Design review of the part built by this model. Coordinates are the model's own, in mm. A direction names the side the tool comes from. Give positions to 0.01 mm unless a question says otherwise; leave off trailing zeros. Write each loop counter-clockwise with the first axis right and the second up, starting at its lowest first coordinate (ties: lowest second). Pieces come first, ordered by that corner, then holes. Notation, with made-up numbers: M 67,43 L 90,43 A15 cw 90,60 Z; hole C 77.25,36.5 d6. An arc over 180 degrees is marked long. One line per item, written item: value. Start each with the question number.
```python
from build123d import *

# Parameters (mm, degrees)
SKETCH2_W           = 280
SKETCH2_H           = 12
SKETCH2_R           = 2
BOSS_EXTRUDE1_DEPTH = 4
CUT_EXTRUDE1_DEPTH  = 281
SKETCH5_R           = 2
BOSS_EXTRUDE2_DEPTH = 2
SKETCH4_W           = 18
SKETCH4_H           = 12
CUT_EXTRUDE2_DEPTH  = 9
BOSS_EXTRUDE3_REACH = 10
SKETCH7_R           = 2
SKETCH8_R           = 2
SKETCH8_R_2         = 1.5
BOSS_EXTRUDE4_DEPTH = 2


with BuildPart() as part:
    # Sketch2 → Boss-Extrude1 (new body, symmetric)
    with BuildSketch(Plane(origin=(0, 0, 0), x_dir=(1, 0, 0), z_dir=(0, 1, 0))):
        Rectangle(SKETCH2_W, SKETCH2_H)
        with Locations((-125, 0)):
            Circle(SKETCH2_R, mode=Mode.SUBTRACT)
        with Locations((-75, 0)):
            Circle(SKETCH2_R, mode=Mode.SUBTRACT)
        with Locations((-25, 0)):
            Circle(SKETCH2_R, mode=Mode.SUBTRACT)
        with Locations((25, 0)):
            Circle(SKETCH2_R, mode=Mode.SUBTRACT)
        with Locations((75, 0)):
            Circle(SKETCH2_R, mode=Mode.SUBTRACT)
        with Locations((125, 0)):
            Circle(SKETCH2_R, mode=Mode.SUBTRACT)
    extrude(amount=BOSS_EXTRUDE1_DEPTH, both=True)

    # Sketch3 → Cut-Extrude1 (cut, through all)
    with BuildSketch(Plane.ZY.offset(140)):
        Polygon((-6, 2.625), (-6, 0.375), (-4.5, 1), (-4.5, 2), align=None)
        Polygon((6, 2.625), (6, 0.375), (4.5, 1), (4.5, 2), align=None)
    extrude(amount=-CUT_EXTRUDE1_DEPTH, mode=Mode.SUBTRACT)

    # Sketch5 → Boss-Extrude2 (add)
    with BuildSketch(Plane(origin=(0, 4, 0), x_dir=(1, 0, 0), z_dir=(0, 1, 0))):
        with Locations((-75, 0)):
            Circle(SKETCH5_R)
        with Locations((-25, 0)):
            Circle(SKETCH5_R)
        with Locations((25, 0)):
            Circle(SKETCH5_R)
        with Locations((75, 0)):
            Circle(SKETCH5_R)
        with Locations((-125, 0)):
            Circle(SKETCH5_R)
        with Locations((125, 0)):
            Circle(SKETCH5_R)
    extrude(amount=-BOSS_EXTRUDE2_DEPTH)

    # Sketch4 → Cut-Extrude2 (cut, through all)
    with BuildSketch(Plane(origin=(0, 4, 0), x_dir=(1, 0, 0), z_dir=(0, 1, 0))):
        with Locations((-131, 0)):
            Rectangle(SKETCH4_W, SKETCH4_H)
    cut_extrude2 = extrude(amount=-CUT_EXTRUDE2_DEPTH, mode=Mode.SUBTRACT)

    # Mirror1: Cut-Extrude2 across plane
    add(cut_extrude2.mirror(Plane(origin=(0, 0, 0), x_dir=(0, 0, 1), z_dir=(1, 0, 0))), mode=Mode.SUBTRACT)

    # Sketch7 → Boss-Extrude3 (add, up to next)
    with BuildSketch(Plane.XZ.offset(4), mode=Mode.PRIVATE) as boss_extrude3_sk1:
        with Locations((-75, 0)):
            Circle(SKETCH7_R)
    boss_extrude3_tool1 = extrude(boss_extrude3_sk1.sketch, amount=-BOSS_EXTRUDE3_REACH, mode=Mode.PRIVATE) - part.part
    add(boss_extrude3_tool1.solids().sort_by_distance((-75, -4, 0))[0])
    # Sketch7 → Boss-Extrude3 (add, up to next)
    with BuildSketch(Plane.XZ.offset(4), mode=Mode.PRIVATE) as boss_extrude3_sk2:
        with Locations((75, 0)):
            Circle(SKETCH7_R)
    boss_extrude3_tool2 = extrude(boss_extrude3_sk2.sketch, amount=-BOSS_EXTRUDE3_REACH, mode=Mode.PRIVATE) - part.part
    add(boss_extrude3_tool2.solids().sort_by_distance((75, -4, 0))[0])

    # Sketch8 → Boss-Extrude4 (add)
    with BuildSketch(Plane.XZ.offset(-2)):
        with Locations((-25, 0)):
            Circle(SKETCH8_R)
        with Locations((-25, 0)):
            Circle(SKETCH8_R_2, mode=Mode.SUBTRACT)
        with Locations((25, 0)):
            Circle(SKETCH8_R)
        with Locations((25, 0)):
            Circle(SKETCH8_R_2, mode=Mode.SUBTRACT)
    extrude(amount=BOSS_EXTRUDE4_DEPTH)


solid = part.part
```
Q1. The part is to be moulded in two halves that separate along X. For faces 1 (the face through (-2, -2, -6)), 2 (the face through (122, 0, 0)), 3 (the face through (-27, -2, 0)), say which applies: pulls with the +X half, pulls with the -X half, needs draft (parallel to the pull), parting line crosses it, or undercut.
Q2. Take a section at A-A, the plane x = 57.5. Give the boundary of the cut face in (y, z) (3 decimals).
Q3. For P1, Ø1.2, axis at x = -25, z = -0.5, coming from the -Y side; P2, Ø0.8, axis at x = 60.5, y = 1.5, coming from the +Z side; P3, Ø0.8, axis at x = -39.5, y = 1.5, coming from the -Z side, all flat-tipped, find the tip position at first contact; note any pin that passes through.
Q4. Wall thickness on line 1 (X direction, y = -2, z = 0); line 2 (Z direction, x = -25, y = 1.65); line 3 (Z direction, x = -25, y = -2.2): over which ranges is each line inside the solid? List them lowest first. Write a range as from..to.
Q5. Machinability: for faces 4 (the face through (23, -2, 0)), 5 (the face through (-2, 4, 0)), which of the approach directions +Z, -Z, +X, -X, +Y, -Y give a long, thin tool a straight path to every point of the face, cutting with its end or side? Answer none if there is none.
Results list:
1. face 1: needs draft
1. face 2: pulls with the +X half
1. face 3: undercut
2. outline: M -4,-6 L 0.375,-6 L 1,-4.5 L 2,-4.5 L 2.625,-6 L 4,-6 L 4,6 L 2.625,6 L 2,4.5 L 1,4.5 L 0.375,6 L -4,6 Z
3. P1: stops at y = 2
3. P2: stops at z = 4.5
3. P3: stops at z = -4.5
4. line 1: x = -122..-27, -23..23, 27..122
4. line 2: z = -4.5..-1.5, 1.5..4.5
4. line 3: z = -6..-2, 2..6
5. face 4: -Y
5. face 5: +Z, -Z, +X, -X, +Y
